Work out the finished part from the listing and answer in its coordinate system (mm). A direction names the side the tool comes from. Coordinates: 2 decimals unless noted, no trailing zeros. Loops run counter-clockwise (first coordinate to the right, second up) from the corner with the lowest first, then second, coordinate; pieces in that order, holes last. Notation, with made-up numbers: (-23.75, 56) -> (13.25, 56) arc R28 ccw to (13.25, 84) -> close; hole circle Ø3 at (6, 86.5). An arc over 180 degrees is marked (long way). Use a Markdown table: item, result. Add a question column.
```python
from build123d import *

# Parameters (mm, degrees)
F1_DEPTH = 63.5
F2_W     = 38.1
F2_H     = 12.702099
F3_DEPTH = 127
F4_R     = 9.525
F4_R_2   = 9.533011
F5_DEPTH = 38.1


with BuildPart() as f1:
    # F0 (on Front) → F1 (new body)
    with BuildSketch(Plane.XZ):
        Polygon((-63.5, 0), (0, 0), (63.5, 0), (63.5, 38.135472), (50.8, 38.135472), (50.8, 25.426184), (0, 25.426184), (-50.8, 25.426184), (-50.8, 38.135472), (-63.5, 38.135472), align=None)
    extrude(amount=F1_DEPTH)

    # F2 (on face) → F3 (cut)
    with BuildSketch(Plane.YZ.offset(63.5)):
        with Locations((-31.760516, 6.351049)):
            Rectangle(F2_W, F2_H)
    extrude(amount=-F3_DEPTH, mode=Mode.SUBTRACT)

    # F4 (on face) → F5 (cut)
    with BuildSketch(Plane.XY.offset(25.426184)):
        with Locations((-19.06892, -31.762339)):
            Circle(F4_R)
        with Locations((19.041387, -31.762339)):
            Circle(F4_R_2)
    extrude(amount=-F5_DEPTH, mode=Mode.SUBTRACT)


solid = f1.part
```
Item 1: Section C-C (y = -58.5) is taken. Determine the outline of the cut face in (x, z).
Item 2: For faces 5 (the face through (1, -31, 25.426)), 6 (the face through (57, -31, 38.135)), 7 (the face through (1, -32, 12.702)), determine the directions among +Z, -Z, +X, -X, +Y, -Y from which every point of the face is accessible in a straight line to the end or side of a thin tool.
Item 3: Section B-B (x = 45) is taken. Determine the outline of the cut face in (y, z).
Item 4: Given pin 1 (22 mm diameter, centred on x = -19.07, y = -31.76, fed in from -Z); pin 2 (11.5 mm diameter, centred on x = 19.04, y = -31.76, fed in from +Z), each flat-ended and moving along its own axis, determine where each tip first touches the part or whether it passes through.
Item 5: Find the intervals of material crossed by probe 1 along Y at (x, z) = (47, 9.5); probe 2 along X at (y, z) = (-40.5, 33.5); probe 3 along Z at (x, y) = (-17, -42.5), in increasing order.
Item 6: Section A-A (z = 27.5) is taken. Determine the outline of the cut face in (x, y).
Item 7: Section D-D (x = 25.5) is taken. Determine the outline of the cut face in (y, z).
Item 8: For a pull along Y with two mould halves and no side action, classify faces 1 (the face through (1, -50.811, 6)), 2 (the face through (-1, -63.5, 15)), 3 (the face through (1, -12.711, 6)), 4 (the face through (-57, -31, 38.135)) as +Y half, -Y half, draft (parallel to the pull), parting line (faces both ways), or undercut.
Output:
| question | item | result |
|---|---|---|
| 1 | outline | (-63.5, 0) -> (63.5, 0) -> (63.5, 38.14) -> (50.8, 38.14) -> (50.8, 25.43) -> (-50.8, 25.43) -> (-50.8, 38.14) -> (-63.5, 38.14) -> close |
| 2 | face 5 | +Z, +Y, -Y |
| 2 | face 6 | +Z, +X, -X, +Y, -Y |
| 2 | face 7 | -Z, +X, -X |
| 3 | outline | (-63.5, 0) -> (-50.81, 0) -> (-50.81, 12.7) -> (-12.71, 12.7) -> (-12.71, 0) -> (0, 0) -> (0, 25.43) -> (-63.5, 25.43) -> close |
| 4 | pin 1 | stops at z = 12.7 |
| 4 | pin 2 | passes through |
| 5 | probe 1 | y = -63.5 to -50.81, -12.71 to 0 |
| 5 | probe 2 | x = -63.5 to -50.8, 50.8 to 63.5 |
| 5 | probe 3 | z = 12.7 to 25.43 |
| 6 | outline | (-63.5, -63.5) -> (-50.8, -63.5) -> (-50.8, 0) -> (-63.5, 0) -> close; (50.8, -63.5) -> (63.5, -63.5) -> (63.5, 0) -> (50.8, 0) -> close |
| 7 | outline | (-63.5, 0) -> (-50.81, 0) -> (-50.81, 12.7) -> (-38.77, 12.7) -> (-38.77, 25.43) -> (-63.5, 25.43) -> close; (-24.75, 12.7) -> (-12.71, 12.7) -> (-12.71, 0) -> (0, 0) -> (0, 25.43) -> (-24.75, 25.43) -> close |
| 8 | face 1 | undercut |
| 8 | face 2 | -Y half |
| 8 | face 3 | undercut |
| 8 | face 4 | draft |
